```python
from build123d import *

# Parameters (mm, degrees)
F1_DEPTH = 4.7
F2_R     = 1
F3_R     = 1
F4_R     = 1
F5_R     = 1
F6_R     = 1
F7_R     = 1


with BuildPart() as f1:
    # F0 (on Top) → F1 (new body)
    with BuildSketch(Plane.XY):
        with BuildLine():
            Line((-37.8634879111, 16.5938198038), (-41.3634879111, 16.5938198038))
            add(Edge.make_bspline(
                [(-41.3634879111, 16.5938198038), (-42.3330999579, 8.4070676233), (-34.6984496013, 2.7716392946), (-27.4017257528, 3.6103434673)],
                knots=[0, 0, 0, 0, 19.0657142627, 19.0657142627, 19.0657142627, 19.0657142627], degree=3))
            Line((-27.4017257528, 3.6103434673), (-27.4715846299, -16.8895375016))
            Line((-27.4715846299, -16.8895375016), (-37.4017257528, -16.8895375016))
            Line((-37.4017257528, -16.8895375016), (-37.4017257528, -21.8895375016))
            Line((-37.4017257528, -21.8895375016), (-27.4017257528, -21.8895375016))
            Line((-27.4017257528, -21.8895375016), (-27.4017257528, -27.8969056376))
            Line((-27.4017257528, -27.8969056376), (-22.4017257528, -27.8969056376))
            Line((-22.4017257528, -27.8969056376), (-22.4017257528, -22.8197725782))
            Line((-22.4017257528, -22.8197725782), (-22.4017257528, 3.9038568961))
            add(Edge.make_bspline(
                [(-28.182390092, 8.1103434673), (-23.6468304455, 7.92984111), (-22.4574972274, 4.6390707602), (-22.4017257528, 3.9038568961)],
                knots=[0, 0, 0, 0, 7.1491684465, 7.1491684465, 7.1491684465, 7.1491684465], degree=3))
            add(Edge.make_bspline(
                [(-37.8634879111, 16.5938198038), (-38.2162182752, 11.5384167701), (-34.5331529288, 7.4555239978), (-28.182390092, 8.1103434673)],
                knots=[0, 0, 0, 0, 12.8721803023, 12.8721803023, 12.8721803023, 12.8721803023], degree=3))
        make_face()
        Polygon((6.2742659492, -17.7634215425), (-22.4017257528, -22.8197725782), (-22.4017257528, -27.8969056376), (7.1425068376, -22.6874603076), align=None)
    extrude(amount=F1_DEPTH)

    # F2
    f2_edges = [f1.edges().sort_by_distance(p)[0] for p in [
        (-32.436655, -16.889538, 4.7),
        (-32.436655, -16.889538, 0),
        (-32.401726, -21.889538, 4.7),
        (-32.401726, -21.889538, 0),
    ]]
    fillet(f2_edges, radius=F2_R)

    # F3
    f3_edges = [f1.edges().sort_by_distance(p)[0] for p in [
        (-27.401726, -27.896906, 2.35),
        (-27.401726, 3.610343, 2.35),
    ]]
    fillet(f3_edges, radius=F3_R)

    # F4
    f4_edges = [f1.edges().sort_by_distance(p)[0] for p in [
        (-41.363488, 16.59382, 2.35),
        (-37.863488, 16.59382, 2.35),
    ]]
    fillet(f4_edges, radius=F4_R)

    # F5
    f5_edges = [f1.edges().sort_by_distance(p)[0] for p in [
        (-22.401726, -22.819773, 2.35),
        (6.274266, -17.763422, 2.35),
        (7.142507, -22.68746, 2.35),
        (6.708386, -20.225441, 0),
        (6.708386, -20.225441, 4.7),
    ]]
    fillet(f5_edges, radius=F5_R)

    # F6
    f6_edges = [f1.edges().sort_by_distance(p)[0] for p in [
        (-37.401726, -16.889538, 2.35),
        (-37.401726, -17.182431, 0.292893),
        (-37.401726, -17.182431, 4.407107),
        (-37.401726, -19.389538, 0),
        (-37.401726, -19.389538, 4.7),
        (-37.401726, -21.596644, 0.292893),
        (-37.401726, -21.596644, 4.407107),
        (-37.401726, -21.889538, 2.35),
    ]]
    fillet(f6_edges, radius=F6_R)

    # F7
    f7_edges = [f1.edges().sort_by_distance(p)[0] for p in [
        (-22.401726, -27.896906, 2.35),
    ]]
    fillet(f7_edges, radius=F7_R)


solid = f1.part
```
Here's how the part is built. I have some questions about the finished solid (model axes, mm). A direction names the side the tool comes from. Give positions to 0.01 mm unless a question says otherwise; leave off trailing zeros. Write each loop counter-clockwise with the first axis right and the second up, starting at its lowest first coordinate (ties: lowest second). Pieces come first, ordered by that corner, then holes. Notation, with made-up numbers: (89.25, 33) -> (111.25, 33) arc R18 ccw to (111.25, 60) -> close; hole circle Ø4 at (68.5, -35.5). An arc over 180 degrees is marked (long way). Write each question's results on one line, items separated by ' | '.
Item 1: Suppose I cut it at A-A on x = 3.5. Write out the boundary of the cut face in (y, z), plus the area to 3 significant figures.
Output:
outline: (-23.33, 0) -> (-18.25, 0) -> (-18.25, 4.7) -> (-23.33, 4.7) -> close | area: 23.9 mm^2
Item 2: If I drill on L1, parallel to X at y = -13.5, z = 4.55; L2, parallel to X at y = 2.5, z = 2.8; L3, parallel to Y at x = 1, z = 0.8, over which ranges is the centre line in solid material (lowest first)?
Output:
L1: x = -27.46 to -22.4 | L2: x = -27.41 to -22.4 | L3: y = -23.77 to -18.69
Item 3: Suppose I cut it at B-B on y = -13.5. Write out the boundary of the cut face in (x, z), plus the area to 3 significant figures.
Output:
outline: (-27.46, 0) -> (-22.4, 0) -> (-22.4, 4.7) -> (-27.46, 4.7) -> close | area: 23.8 mm^2
Item 4: We'd pull the mould along X, two halves only. Please class faces 1 (the face through (-7.78, -20.24, 2.32)), 2 (the face through (-22.05, -22.39, 2.38)), 3 (the face through (-32, -16.89, 2)), 4 (the face through (-37.117, -21.589, 2.331)): pulls with the +X half, pulls with the -X half, needs draft (parallel to the pull), parting line crosses it, or undercut.
Output:
face 1: undercut | face 2: undercut | face 3: needs draft | face 4: pulls with the -X half
Item 5: For pin 1 Ø2.5 at (y, z) = (-22.5, 3) entering from -X; pin 2 Ø1.4 at (y, z) = (-19.5, 2.5) entering from -X; pin 3 Ø2 at (x, z) = (-17, 0.5) entering from -Y, each with a flat end and sliding along its axis, tell me the tip position at first contact or that it passes through.
Output:
pin 1: stops at x = -37.33 | pin 2: stops at x = -37.4 | pin 3: stops at y = -27.12
Item 6: On a 3-axis mill with a long thin cutter (end or side, diameter ignored), from which of +Z, -Z, +X, -X, +Y, -Y can I reach the whole of each face in a straight line? I mean faces 5 (the face through (-31.839, -21.604, 4.399)), 6 (the face through (-37.117, -19.369, 0.301)), 7 (the face through (-37.402, -19, 2)). Say none if no direction works.
Output:
face 5: +Z, -X, -Y | face 6: -Z, -X, -Y | face 7: +Z, -Z, -X, -Y
